For this review, take the finished solid that the model builds, in its own axes (mm). A direction names the side the tool comes from. Give positions to 0.01 mm unless a question says otherwise; leave off trailing zeros. Write each loop counter-clockwise with the first axis right and the second up, starting at its lowest first coordinate (ties: lowest second). Pieces come first, ordered by that corner, then holes.
Q1. We need section C-C (y = 6.75). Write out the cut boundary in (x, z), then the cut area to 3 significant figures.
Q2. Mouldability with a two-part tool opening along Z and no side actions: class faces 1 (the flat face through (1, 8, 40)), 2 (the cylindrical face through (6.93, -2.87, 19.72)), 3 (the flat face through (-8, 0, 14.5)) as released by +Z, released by -Z, zero draft, split by the parting line, or undercut.
Q3. Insertion check: P1, Ø1.5, axis at x = -5.5, z = 19, coming from the +Y side; P2, Ø2.5, axis at x = -8, z = 22, coming from the +Y side; P3, Ø2, axis at x = -5, z = 12.5, coming from the -Y side. Each pin has a flat end and moves straight along its axis. Give the tip position at first contact, or say it passes through.
Q4. For line 1 (Y direction, x = 0, z = 18); line 2 (Y direction, x = 4.5, z = 32); line 3 (X direction, y = -2.5, z = 34.5), list the stretches that pass through material, from the lowest coordinate up.
Q5. We need section D-D (z = 28.5). Write out the cut boundary in (x, y), then the cut area to 3 significant figures.
Q6. Machinability: for faces 4 (the flat face through (1, 8, 0)), 5 (the flat face through (-8, 0, 25.5)), which of the approach directions +Z, -Z, +X, -X, +Y, -Y give a long, thin tool a straight path to every point of the face, cutting with its end or side? Answer none if there is none.
Q7. We need section A-A (y = 0). Write out the cut boundary in (x, z), then the cut area to 3 significant figures.
Q8. We need section B-B (x = 0). Write out the cut boundary in (y, z), then the cut area to 3 significant figures.
```python
from build123d import *

# Parameters (mm, degrees)
F0_R     = 9.5
F0_R_2   = 7.5
F1_DEPTH = 40
F2_W     = 5
F2_H     = 11
F3_DEPTH = 25


with BuildPart() as f1:
    # F0 (on Top) → F1 (new body)
    with BuildSketch(Plane.XY):
        Circle(F0_R)
        Circle(F0_R_2, mode=Mode.SUBTRACT)
    extrude(amount=F1_DEPTH)

    # F2 (on Right) → F3 (cut)
    with BuildSketch(Plane.YZ):
        with Locations((0, 20)):
            Rectangle(F2_W, F2_H)
    extrude(amount=-F3_DEPTH, mode=Mode.SUBTRACT)


solid = f1.part
```
Computed:
1. outline: (-6.68, 0) - (-3.27, 0) - (-3.27, 40) - (-6.68, 40) - close; (3.27, 0) - (6.68, 0) - (6.68, 40) - (3.27, 40) - close
1. area: 273 mm2
2. face 1: released by +Z
2. face 2: zero draft
2. face 3: undercut
3. P1: stops at y = 8.23
3. P2: stops at y = 6.68
3. P3: stops at y = -8.62
4. line 1: y = -9.5 to -7.5, 7.5 to 9.5
4. line 2: y = -8.37 to -6, 6 to 8.37
4. line 3: x = -9.17 to -7.07, 7.07 to 9.17
5. outline: circle Ø19 at (0, 0); hole circle Ø15 at (0, 0)
5. area: 107 mm2
6. face 4: -Z, +X, -X, +Y, -Y
6. face 5: -X
7. outline: (-9.5, 0) - (-7.5, 0) - (-7.5, 14.5) - (-9.5, 14.5) - close; (-9.5, 25.5) - (-7.5, 25.5) - (-7.5, 40) - (-9.5, 40) - close; (7.5, 0) - (9.5, 0) - (9.5, 40) - (7.5, 40) - close
7. area: 138 mm2
8. outline: (-9.5, 0) - (-7.5, 0) - (-7.5, 40) - (-9.5, 40) - close; (7.5, 0) - (9.5, 0) - (9.5, 40) - (7.5, 40) - close
8. area: 160 mm2
